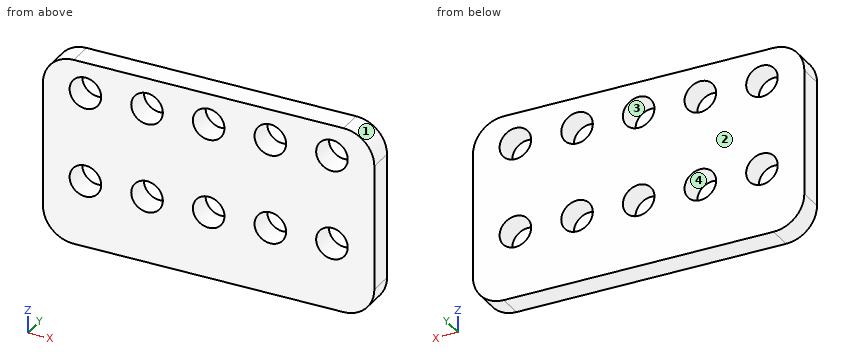
```python
from build123d import *

# Parameters (mm, degrees)
SKETCH1_W           = 43
SKETCH1_H           = 24.3
SKETCH1_R           = 2.05
BOSS_EXTRUDE1_DEPTH = 3.175
FILLET1_R           = 4


with BuildPart() as part:
    # Sketch1 → Boss-Extrude1 (new body)
    with BuildSketch(Plane(origin=(0, 0, 0), x_dir=(1, 0, 0), z_dir=(0, 1, 0))):
        Rectangle(SKETCH1_W, SKETCH1_H)
        with Locations(Location((-16, -8.15, 0), (0, 0, 270))):
            Circle(SKETCH1_R, mode=Mode.SUBTRACT)
        with Locations(Location((-8, -8.15, 0), (0, 0, 270))):
            Circle(SKETCH1_R, mode=Mode.SUBTRACT)
        with Locations(Location((0, -8.15, 0), (0, 0, 270))):
            Circle(SKETCH1_R, mode=Mode.SUBTRACT)
        with Locations(Location((8, -8.15, 0), (0, 0, 270))):
            Circle(SKETCH1_R, mode=Mode.SUBTRACT)
        with Locations(Location((16, -8.15, 0), (0, 0, 270))):
            Circle(SKETCH1_R, mode=Mode.SUBTRACT)
        with Locations(Location((-16, 3.47, 0), (0, 0, 270))):
            Circle(SKETCH1_R, mode=Mode.SUBTRACT)
        with Locations(Location((-8, 3.47, 0), (0, 0, 270))):
            Circle(SKETCH1_R, mode=Mode.SUBTRACT)
        with Locations(Location((0, 3.47, 0), (0, 0, 270))):
            Circle(SKETCH1_R, mode=Mode.SUBTRACT)
        with Locations(Location((8, 3.47, 0), (0, 0, 270))):
            Circle(SKETCH1_R, mode=Mode.SUBTRACT)
        with Locations(Location((16, 3.47, 0), (0, 0, 270))):
            Circle(SKETCH1_R, mode=Mode.SUBTRACT)
    extrude(amount=BOSS_EXTRUDE1_DEPTH)

    # Fillet1
    fillet1_edges = [part.edges().sort_by_distance(p)[0] for p in [
        (-21.5, 1.5875, -12.15),
        (21.5, 1.5875, -12.15),
        (21.5, 1.5875, 12.15),
        (-21.5, 1.5875, 12.15),
    ]]
    fillet(fillet1_edges, radius=FILLET1_R)


solid = part.part
```
Can you work these out from the model? Positions are in its coordinate system, mm. Face numbers are marked on the shaded views. Give positions to 0.01 mm unless a question says otherwise; leave off trailing zeros. Write each loop counter-clockwise with the first axis right and the second up, starting at its lowest first coordinate (ties: lowest second). Pieces come first, ordered by that corner, then holes. Notation, with made-up numbers: (-17.75, -11.5) - (-4.75, -11.5) arc R17 ccw to (-4.75, 14.5) - close; hole circle Ø2 at (56, 20.5). An arc over 180 degrees is marked (long way). Write item = value, one per line. Start each with the question number.
1. Thinking about a two-plate mould opening in X: for the marked faces 1, 2, 3 and 4, which applies, released by +X, released by -X, zero draft, split by the parting line, or undercut?
2. Imagine slicing it at C-C (z = -3.75). Please give me the cut outline in (x, y) (3 decimals), and give its area (3 significant figures).
3. Imagine slicing it at B-B (x = -8). Please give me the cut outline in (y, z) (3 decimals).
4. For pin 1 (8 mm diameter, centred on x = -12.5, z = 8.5, fed in from -Y), with a flat end and sliding along its axis, tell me the tip position at first contact or that it passes through.
5. Imagine slicing it at D-D (x = 1.5). Please give me the cut outline in (y, z) (3 decimals).
6. Please list where these lines run through material, in increasing order: line 1 (X direction, y = 3, z = 8); line 2 (Z direction, x = 9.5, y = 0.1); line 3 (X direction, y = 2.9, z = 6.5).
7. Imagine slicing it at A-A (y = 2.7). Count the separate pieces of the cut face and the enclosed holes in it, and give its area (3 significant figures).
Worked answers:
q1.face_1 = released by +X
q1.face_2 = zero draft
q1.face_3 = undercut
q1.face_4 = undercut
q2.outline = (-21.5, 0) - (-18.031, 0) - (-18.031, 3.175) - (-21.5, 3.175) - close; (-13.969, 0) - (-10.031, 0) - (-10.031, 3.175) - (-13.969, 3.175) - close; (-5.969, 0) - (-2.031, 0) - (-2.031, 3.175) - (-5.969, 3.175) - close; (2.031, 0) - (5.969, 0) - (5.969, 3.175) - (2.031, 3.175) - close; (10.031, 0) - (13.969, 0) - (13.969, 3.175) - (10.031, 3.175) - close; (18.031, 0) - (21.5, 0) - (21.5, 3.175) - (18.031, 3.175) - close
q2.area = 72.0 mm2
q3.outline = (0, -12.15) - (3.175, -12.15) - (3.175, -5.52) - (0, -5.52) - close; (0, -1.42) - (3.175, -1.42) - (3.175, 6.1) - (0, 6.1) - close; (0, 10.2) - (3.175, 10.2) - (3.175, 12.15) - (0, 12.15) - close
q4.pin_1 = 0
q5.outline = (0, -12.15) - (3.175, -12.15) - (3.175, -4.867) - (0, -4.867) - close; (0, -2.073) - (3.175, -2.073) - (3.175, 6.753) - (0, 6.753) - close; (0, 9.547) - (3.175, 9.547) - (3.175, 12.15) - (0, 12.15) - close
q6.line_1 = -21.5 to -18.04, -13.96 to -10.04, -5.96 to -2.04, 2.04 to 5.96, 10.04 to 13.96, 18.04 to 21.5
q6.line_2 = -12.15 to -4.87, -2.07 to 6.75, 9.55 to 12.15
q6.line_3 = -21.5 to -17.22, -14.78 to -9.22, -6.78 to -1.22, 1.22 to 6.78, 9.22 to 14.78, 17.22 to 21.5
q7.separate_pieces = 1
q7.enclosed_holes = 10
q7.area = 899 mm2
